from build123d import *

# Parameters (mm, degrees)
ESQUISSE1_R        = 3
BOSS_EXTRU_1_DEPTH = 130


with BuildPart() as part:
    # Esquisse1 → Boss.-Extru.1 (new body)
    with BuildSketch(Plane.XY):
        with BuildLine():
            Line((18.273972397, -2.817988329), (18.273972397, -4.763988771))
            ThreePointArc((18.273972397, -4.763988771), (18.188448617, -4.970461441), (17.981975947, -5.055985222))
            Line((17.981975947, -5.055985222), (16.798674025, -5.055985222))
            ThreePointArc((16.798674025, -5.055985222), (16.686931822, -5.033758315), (16.592201355, -4.970461441))
            Line((16.592201355, -4.970461441), (14.174856283, -2.553116369))
            ThreePointArc((14.174856283, -2.553116369), (14.111559409, -2.458385902), (14.089332502, -2.346643699))
            Line((14.089332502, -2.346643699), (14.089332502, -0.209112213))
            Line((14.089332502, -0.209112213), (13.797336052, 0.296640474))
            Line((13.797336052, 0.296640474), (14.089332502, 0.802393162))
            Line((14.089332502, 0.802393162), (14.089332502, 2.939924647))
            ThreePointArc((14.089332502, 2.939924647), (14.111559409, 3.051666851), (14.174856283, 3.146397317))
            Line((14.174856283, 3.146397317), (16.592201355, 5.56374239))
            ThreePointArc((16.592201355, 5.56374239), (16.686931822, 5.627039264), (16.798674025, 5.64926617))
            Line((16.798674025, 5.64926617), (17.981975947, 5.64926617))
            ThreePointArc((17.981975947, 5.64926617), (18.188448617, 5.56374239), (18.273972397, 5.35726972))
            Line((18.273972397, 5.35726972), (18.273972397, 3.411269278))
            ThreePointArc((18.273972397, 3.411269278), (18.334057146, 3.321346096), (18.440128771, 3.342445054))
            Line((18.440128771, 3.342445054), (19.940427319, 4.842743602))
            ThreePointArc((19.940427319, 4.842743602), (20.003724193, 4.937474069), (20.025951099, 5.049216272))
            Line((20.025951099, 5.049216272), (20.025951099, 9.737859034))
            ThreePointArc((20.025951099, 9.737859034), (19.940427319, 9.944331704), (19.733954649, 10.029855484))
            Line((19.733954649, 10.029855484), (15.045311887, 10.029855484))
            ThreePointArc((15.045311887, 10.029855484), (14.933569683, 10.007628578), (14.838839217, 9.944331704))
            Line((14.838839217, 9.944331704), (13.338540669, 8.444033156))
            ThreePointArc((13.338540669, 8.444033156), (13.317441711, 8.337961531), (13.407364892, 8.277876782))
            Line((13.407364892, 8.277876782), (15.353365335, 8.277876782))
            ThreePointArc((15.353365335, 8.277876782), (15.559838005, 8.192353002), (15.645361785, 7.985880332))
            Line((15.645361785, 7.985880332), (15.645361785, 6.802578411))
            ThreePointArc((15.645361785, 6.802578411), (15.623134879, 6.690836207), (15.559838005, 6.596105741))
            Line((15.559838005, 6.596105741), (13.142492932, 4.178760668))
            ThreePointArc((13.142492932, 4.178760668), (13.047762466, 4.115463794), (12.936020262, 4.093236888))
            Line((12.936020262, 4.093236888), (10.798488777, 4.093236888))
            Line((10.798488777, 4.093236888), (10.292736089, 3.801240437))
            Line((10.292736089, 3.801240437), (9.786983402, 4.093236888))
            Line((9.786983402, 4.093236888), (7.649451916, 4.093236888))
            ThreePointArc((7.649451916, 4.093236888), (7.537709712, 4.115463794), (7.442979246, 4.178760668))
            Line((7.442979246, 4.178760668), (5.025634173, 6.596105741))
            ThreePointArc((5.025634173, 6.596105741), (4.962337299, 6.690836207), (4.940110393, 6.802578411))
            Line((4.940110393, 6.802578411), (4.940110393, 7.985880332))
            ThreePointArc((4.940110393, 7.985880332), (5.025634173, 8.192353002), (5.232106843, 8.277876782))
            Line((5.232106843, 8.277876782), (7.178107286, 8.277876782))
            ThreePointArc((7.178107286, 8.277876782), (7.268030467, 8.337961531), (7.246931509, 8.444033156))
            Line((7.246931509, 8.444033156), (5.746632961, 9.944331704))
            ThreePointArc((5.746632961, 9.944331704), (5.651902495, 10.007628578), (5.540160291, 10.029855484))
            Line((5.540160291, 10.029855484), (0.85151753, 10.029855484))
            ThreePointArc((0.85151753, 10.029855484), (0.64504486, 9.944331704), (0.559521079, 9.737859034))
            Line((0.559521079, 9.737859034), (0.559521079, 5.049216272))
            ThreePointArc((0.559521079, 5.049216272), (0.581747986, 4.937474069), (0.64504486, 4.842743602))
            Line((0.64504486, 4.842743602), (2.145343408, 3.342445054))
            ThreePointArc((2.145343408, 3.342445054), (2.251415032, 3.321346096), (2.311499781, 3.411269278))
            Line((2.311499781, 3.411269278), (2.311499781, 5.35726972))
            ThreePointArc((2.311499781, 5.35726972), (2.397023561, 5.56374239), (2.603496231, 5.64926617))
            Line((2.603496231, 5.64926617), (3.786798153, 5.64926617))
            ThreePointArc((3.786798153, 5.64926617), (3.898540357, 5.627039264), (3.993270823, 5.56374239))
            Line((3.993270823, 5.56374239), (6.410615896, 3.146397317))
            ThreePointArc((6.410615896, 3.146397317), (6.47391277, 3.051666851), (6.496139676, 2.939924647))
            Line((6.496139676, 2.939924647), (6.496139676, 0.802393162))
            Line((6.496139676, 0.802393162), (6.788136126, 0.296640474))
            Line((6.788136126, 0.296640474), (6.496139676, -0.209112213))
            Line((6.496139676, -0.209112213), (6.496139676, -2.346643699))
            ThreePointArc((6.496139676, -2.346643699), (6.47391277, -2.458385902), (6.410615896, -2.553116369))
            Line((6.410615896, -2.553116369), (3.993270823, -4.970461441))
            ThreePointArc((3.993270823, -4.970461441), (3.898540357, -5.033758315), (3.786798153, -5.055985222))
            Line((3.786798153, -5.055985222), (2.603496231, -5.055985222))
            ThreePointArc((2.603496231, -5.055985222), (2.397023561, -4.970461441), (2.311499781, -4.763988771))
            Line((2.311499781, -4.763988771), (2.311499781, -2.817988329))
            ThreePointArc((2.311499781, -2.817988329), (2.251415032, -2.728065147), (2.145343408, -2.749164105))
            Line((2.145343408, -2.749164105), (0.64504486, -4.249462653))
            ThreePointArc((0.64504486, -4.249462653), (0.581747986, -4.34419312), (0.559521079, -4.455935324))
            Line((0.559521079, -4.455935324), (0.559521079, -9.144578085))
            ThreePointArc((0.559521079, -9.144578085), (0.64504486, -9.351050755), (0.85151753, -9.436574535))
            Line((0.85151753, -9.436574535), (5.540160291, -9.436574535))
            ThreePointArc((5.540160291, -9.436574535), (5.651902495, -9.414347629), (5.746632961, -9.351050755))
            Line((5.746632961, -9.351050755), (7.246931509, -7.850752207))
            ThreePointArc((7.246931509, -7.850752207), (7.268030467, -7.744680582), (7.178107286, -7.684595834))
            Line((7.178107286, -7.684595834), (5.232106843, -7.684595834))
            ThreePointArc((5.232106843, -7.684595834), (5.025634173, -7.599072053), (4.940110393, -7.392599383))
            Line((4.940110393, -7.392599383), (4.940110393, -6.209297462))
            ThreePointArc((4.940110393, -6.209297462), (4.962337299, -6.097555258), (5.025634173, -6.002824792))
            Line((5.025634173, -6.002824792), (7.442979246, -3.585479719))
            ThreePointArc((7.442979246, -3.585479719), (7.537709712, -3.522182845), (7.649451916, -3.499955939))
            Line((7.649451916, -3.499955939), (9.786983402, -3.499955939))
            Line((9.786983402, -3.499955939), (10.292736089, -3.207959489))
            Line((10.292736089, -3.207959489), (10.798488777, -3.499955939))
            Line((10.798488777, -3.499955939), (12.936020262, -3.499955939))
            ThreePointArc((12.936020262, -3.499955939), (13.047762466, -3.522182845), (13.142492932, -3.585479719))
            Line((13.142492932, -3.585479719), (15.559838005, -6.002824792))
            ThreePointArc((15.559838005, -6.002824792), (15.623134879, -6.097555258), (15.645361785, -6.209297462))
            Line((15.645361785, -6.209297462), (15.645361785, -7.392599383))
            ThreePointArc((15.645361785, -7.392599383), (15.559838005, -7.599072053), (15.353365335, -7.684595834))
            Line((15.353365335, -7.684595834), (13.407364892, -7.684595834))
            ThreePointArc((13.407364892, -7.684595834), (13.317441711, -7.744680582), (13.338540669, -7.850752207))
            Line((13.338540669, -7.850752207), (14.838839217, -9.351050755))
            ThreePointArc((14.838839217, -9.351050755), (14.933569683, -9.414347629), (15.045311887, -9.436574535))
            Line((15.045311887, -9.436574535), (19.733954649, -9.436574535))
            ThreePointArc((19.733954649, -9.436574535), (19.940427319, -9.351050755), (20.025951099, -9.144578085))
            Line((20.025951099, -9.144578085), (20.025951099, -4.455935324))
            ThreePointArc((20.025951099, -4.455935324), (20.003724193, -4.34419312), (19.940427319, -4.249462653))
            Line((19.940427319, -4.249462653), (18.440128771, -2.749164105))
            ThreePointArc((18.440128771, -2.749164105), (18.334057146, -2.728065147), (18.273972397, -2.817988329))
        make_face()
        with Locations((10.292736089, 0.296640474)):
            Circle(ESQUISSE1_R, mode=Mode.SUBTRACT)
    extrude(amount=BOSS_EXTRU_1_DEPTH)


solid = part.part
Work out the finished part from the listing and answer in its coordinate system (mm). A direction names the side the tool comes from. Coordinates: 2 decimals unless noted, no trailing zeros. Answer as CSV lines item,"result". Start each with the question number.
Item 1: Flat-ended cylindrical pins translate along their axes: P1, Ø1.7, axis at x = 8, z = 94.5, coming from the -Y side; P2, Ø1.6, axis at y = -3.5, z = 91.5, coming from the -X side; P3, Ø1, axis at y = -3.5, z = 90.5, coming from the +X side. Find the tip coordinate at first contact, or state that the pin passes through.
Item 2: Consider L1, parallel to Y at x = 13.75, z = 95; L2, parallel to X at y = -4.5, z = 122; L3, parallel to Y at x = 16.75, z = 73. Determine where each line is inside the solid, lowest interval first.
Item 3: A tool of negligible diameter and unlimited length cuts with its end or side. For faces 1 (the face through (3, 10.03, 64)), 2 (the face through (17, -9.437, 64)), 3 (the face through (15.4, -3.78, 64.09)), 4 (the face through (12, 4.093, 64)), 5 (the face through (14.089, -1, 64)), from which of +Z, -Z, +X, -X, +Y, -Y can it reach the whole face along a straight path? Write none if from no direction.
Item 4: Determine the mould class of faces 6 (the face through (14.089, 2, 64)), 7 (the face through (3, -9.437, 64)), 8 (the face through (9, -3.5, 64)) for opening direction X: released by +X, released by -X, zero draft, split by the parting line, or undercut.
Checks:
1,P1,"stops at y = -7.95"
1,P2,"stops at x = 0.6"
1,P3,"stops at x = 19.69"
2,L1,"y = -8.26 to -7.68, -4.19 to 4.79, 8.28 to 8.86"
2,L2,"x = 0.56 to 2.31, 4.46 to 6.53, 14.06 to 16.12, 18.27 to 20.03"
2,L3,"y = -9.44 to -5.05, 5.65 to 10.03"
3,face 1,"+Z, -Z, +X, -X, +Y"
3,face 2,"+Z, -Z, +X, -X, -Y"
3,face 3,"+Z, -Z"
3,face 4,"+Z, -Z, +Y"
3,face 5,"+Z, -Z, +X"
4,face 6,"released by +X"
4,face 7,"zero draft"
4,face 8,"undercut"
